Source: CAD feature listing. Evaluate the final solid. Frame: model axes, mm. Face numbers are marked on the shaded views. A direction names the side the tool comes from. Give positions to 0.01 mm unless a question says otherwise; leave off trailing zeros. Loops run counter-clockwise (first coordinate to the right, second up) from the corner with the lowest first, then second, coordinate; pieces in that order, holes last. Notation, with made-up numbers: M -16,27.25 L -10,27.25 A19 cw -10,34.25 Z; hole C 55,-20.5 d10. An arc over 180 degrees is marked long. Answer in a Markdown table with one row per item.
```python
from build123d import *

# Parameters (mm, degrees)
SKETCH1_R           = 28.5
BOSS_EXTRUDE1_DEPTH = 10.5
SHELL1_OUTLINE_R    = 27.5
SHELL1_DEPTH        = 7.5
CUT_EXTRUDE3_DEPTH  = 9.5
CUT_EXTRUDE4_DEPTH  = 42.409539964
CUT_EXTRUDE2_START  = -2
CUT_EXTRUDE2_DEPTH  = 2
CIRPATTERN1_COUNT   = 4
CHAMFER2_SIZE       = 1
CUT_EXTRUDE5_DEPTH  = 0.8
CHAMFER3_SIZE       = 1


with BuildPart() as part:
    # Sketch1 → Boss-Extrude1 (new body)
    with BuildSketch(Plane(origin=(0, 0, 0), x_dir=(1, 0, 0), z_dir=(0, 1, 0))):
        with Locations(Location((0, 0, 0), (0, 0, 90))):
            Circle(SKETCH1_R)
    extrude(amount=BOSS_EXTRUDE1_DEPTH)

    # Shell1: read off the stored shape, not the designer's step
    # Shell1 outline → Shell1 (cut)
    with BuildSketch(Plane(origin=(0, 0, 0), x_dir=(1, 0, 0), z_dir=(0, 1, 0))):
        Circle(SHELL1_OUTLINE_R)
    extrude(amount=SHELL1_DEPTH, mode=Mode.SUBTRACT)

    # Sketch6 → Cut-Extrude3 (cut)
    with BuildSketch(Plane.XZ):
        with BuildLine():
            Line((16, 28.5), (16, 15.81929202))
            ThreePointArc((16, 15.81929202), (0, -22.5), (-16, 15.81929202))
            Line((-16, 15.81929202), (-16, 28.5))
            Line((-16, 28.5), (16, 28.5))
        make_face()
    extrude(amount=-CUT_EXTRUDE3_DEPTH, mode=Mode.SUBTRACT)

    # Sketch7 → Cut-Extrude4 (cut, through all)
    with BuildSketch(Plane.XZ.offset(-9.5)):
        with BuildLine():
            Line((-16, 23.58495283), (16, 23.58495283))
            ThreePointArc((16, 23.58495283), (0, 28.5), (-16, 23.58495283))
        make_face()
    extrude(amount=-CUT_EXTRUDE4_DEPTH, mode=Mode.SUBTRACT)

    # Sketch3 → Cut-Extrude2 (cut)
    with BuildSketch(Plane(origin=(0, 10.5, 0), x_dir=(1, 0, 0), z_dir=(0, 1, 0)).offset(CUT_EXTRUDE2_START)):
        with BuildLine():
            Line((16.970562748, -19.798989873), (18.688646931, -21.517074055))
            ThreePointArc((18.688646931, -21.517074055), (20.152543264, -20.152543264), (21.517074055, -18.688646931))
            Line((21.517074055, -18.688646931), (19.798989873, -16.970562748))
            ThreePointArc((19.798989873, -16.970562748), (16.970562748, -16.970562748), (16.970562748, -19.798989873))
        make_face()
    cut_extrude2 = extrude(amount=CUT_EXTRUDE2_DEPTH, mode=Mode.SUBTRACT)

    # CirPattern1: Cut-Extrude2 ×4 about axis
    cirpattern1_axis = Axis((0, 0, 0), (0, 1, 0))
    for i in range(1, CIRPATTERN1_COUNT):
        add(cut_extrude2.rotate(cirpattern1_axis, i * 360 / CIRPATTERN1_COUNT), mode=Mode.SUBTRACT)

    # Chamfer2
    chamfer2_edges = [part.edges().sort_by_distance(p)[0] for p in [
        (-20.658031964, 10.5, 17.82960484),
        (-16.970562748, 10.5, 16.970562748),
        (-17.82960484, 10.5, 20.658031964),
        (-17.375114018, 10.5, 22.591047184),
        (0, 10.5, 23.58495283),
        (17.375114018, 10.5, 22.591047184),
        (17.82960484, 10.5, 20.658031964),
        (16.970562748, 10.5, 16.970562748),
        (20.658031964, 10.5, 17.82960484),
        (28.5, 10.5, 0),
        (20.658031964, 10.5, -17.82960484),
        (16.970562748, 10.5, -16.970562748),
        (17.82960484, 10.5, -20.658031964),
        (0, 10.5, -28.5),
        (-17.82960484, 10.5, -20.658031964),
        (-16.970562748, 10.5, -16.970562748),
        (-20.658031964, 10.5, -17.82960484),
        (-28.5, 10.5, 0),
    ]]
    chamfer(chamfer2_edges, length=CHAMFER2_SIZE - 0.0001)  # a hair under: the kernel refuses the full size

    # Sketch9 → Cut-Extrude5 (cut)
    with BuildSketch(Plane.XZ.offset(-9.5)):
        with BuildLine():
            Line((-5.5, 23.58495283), (5.5, 23.58495283))
            Line((5.5, 23.58495283), (5.5, 15.58495283))
            ThreePointArc((5.5, 15.58495283), (4.914213562, 14.170739268), (3.5, 13.58495283))
            Line((3.5, 13.58495283), (-3.5, 13.58495283))
            ThreePointArc((-3.5, 13.58495283), (-4.914213562, 14.170739268), (-5.5, 15.58495283))
            Line((-5.5, 15.58495283), (-5.5, 23.58495283))
        make_face()
    extrude(amount=-CUT_EXTRUDE5_DEPTH, mode=Mode.SUBTRACT)

    # Chamfer3
    # the kernel refuses this chamfer: 1, 0.719970543 mm, written as the material it takes off along each edge
    with BuildSketch(Plane(origin=(-16, 9.5, 23.58495283), x_dir=(-0.8204018927518858, 0, -0.5717873156770121), z_dir=(0, -1, 0))) as chamfer3_piece_1:
        with BuildLine():
            Line((0.71829317, 0), (CHAMFER3_SIZE * 0.571787315677, CHAMFER3_SIZE * 0.820401892752))
            Line((CHAMFER3_SIZE * 0.571787315677, CHAMFER3_SIZE * 0.820401892752), (0, 0))
            ThreePointArc((0, 0), (0.362660378, -0.00226279), (0.71829317, 0))
        make_face()
    extrude(amount=12.071682988, mode=Mode.SUBTRACT)
    with BuildSketch(Plane(origin=(16, 9.5, 23.58495283), x_dir=(0.8204018927518871, 0, -0.5717873156770101), z_dir=(0, -1, 0))) as chamfer3_piece_2:
        with BuildLine():
            Line((0.71829317, 0), (CHAMFER3_SIZE * 0.571787315677, -CHAMFER3_SIZE * 0.820401892752))
            Line((CHAMFER3_SIZE * 0.571787315677, -CHAMFER3_SIZE * 0.820401892752), (0, 0))
            ThreePointArc((0, 0), (0.362660378, 0.00226279), (0.71829317, 0))
        make_face()
    extrude(amount=12.071682988, mode=Mode.SUBTRACT)

    # Sketch11 → Cut-Revolve2 (revolve, cut)
    with BuildSketch(Plane.XY):
        Polygon((28, 7), (28, 6.5), (28.5, 6), (28.5, 3.5), (28, 3), (28, 2.5), (28.5, 2), (29.5, 2), (29.5, 7.5), (28.5, 7.5), align=None)
    revolve(axis=Axis((0, 43.121181377, 0), (0, -1, 0)), mode=Mode.SUBTRACT)


solid = part.part
```
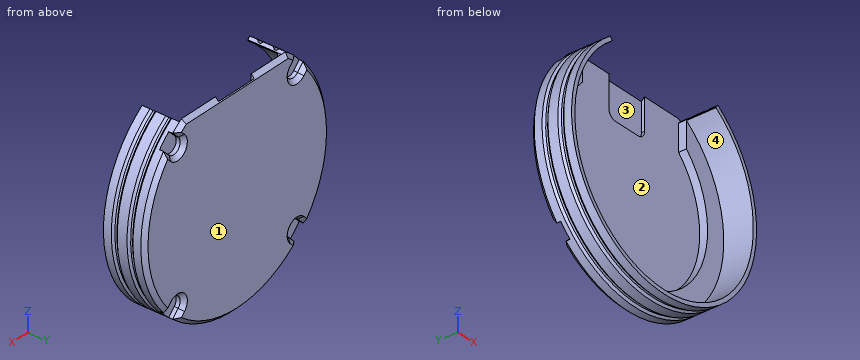
1) Section B-B, the plane x = 0. Return loops of the section in (y, z), then the cut area to 3 significant figures.
Reply:
| item | result |
|---|---|
| outline | M 0,-28.5 L 2,-28.5 L 2.5,-28 L 3,-28 L 3.5,-28.5 L 6,-28.5 L 6.5,-28 L 7,-28 L 7.5,-28.5 L 9.5,-28.5 L 10.5,-27.5 L 10.5,22.59 L 10.3,22.79 L 10.3,13.58 L 9.5,13.58 L 9.5,-22.5 L 7.5,-22.5 L 7.5,-27.5 L 0,-27.5 Z |
| area | 61.9 mm² |
2) Pull-direction query (X, two-part tool) for the marked faces 1 and 2; classes: released by +X, released by -X, zero draft, split by the parting line, or undercut.
Reply:
| item | result |
|---|---|
| face 1 | zero draft |
| face 2 | undercut |
3) Set-up query: the marked faces 3 and 4. Return all of +Z, -Z, +X, -X, +Y, -Y with unobstructed straight access to the full face (end or side cutting, diameter ignored); none if empty.
Reply:
| item | result |
|---|---|
| face 3 | +Z, -Y |
| face 4 | -Y |
4) Material intervals for L1, parallel to X at y = 9, z = -0.5; L2, parallel to X at y = 2.5, z = 0; L3, parallel to Y at x = 17.5, z = -3, sorted ascending.
Reply:
| item | result |
|---|---|
| L1 | x = -28.5 to -22.49, 22.49 to 28.5 |
| L2 | x = -28 to -27.5, 27.5 to 28 |
| L3 | y = 9.5 to 10.5 |
5) Pin query (flat end, axial travel): pin 1 Ø3 at (x, z) = (1, 17.5) entering from -Y; pin 2 Ø5.5 at (x, z) = (-18, -18.5) entering from +Y; pin 3 Ø6 at (y, z) = (2.5, -6.5) entering from -X; pin 4 Ø25 at (x, z) = (8, 9) entering from -Y. Return the tip coordinate at first contact, or that it passes through.
Reply:
| item | result |
|---|---|
| pin 1 | stops at y = 10.3 |
| pin 2 | stops at y = 10.5 |
| pin 3 | stops at x = -28.28 |
| pin 4 | stops at y = 7.5 |
